Read the model definition and answer for the solid it produces. Units are mm, in the model's axes. Coordinates: 2 decimals unless noted, no trailing zeros. Write each loop counter-clockwise with the first axis right and the second up, starting at its lowest first coordinate (ties: lowest second). Pieces come first, ordered by that corner, then holes. Notation, with made-up numbers: (86, 32) - (136, 32) arc R20 cw to (136, 38) - close; hole circle Ø6 at (-34.5, 5.25). An arc over 180 degrees is marked (long way). Use a Markdown table: item, result.
from build123d import *

# Parameters (mm, degrees)
BOSS_EXTRUDE1_DEPTH         = 2.54
F_48_0_076_DIAMETER_HOLE1_D = 1.9304


with BuildPart() as part:
    # Sketch1 → Boss-Extrude1 (new body)
    with BuildSketch(Plane.XY):
        with BuildLine():
            Line((-1.523739013, -6.254008737), (3.199990263, -6.407247691))
            ThreePointArc((3.199990263, -6.407247691), (4.013460409, -6.008075165), (4.137562895, -5.110483411))
            add(Edge.make_bspline(
                [(4.137562895, -5.110483411), (3.751708737, -4.057424722), (1.960352922, -2.838406427), (0.682892057, -0.893226264), (0.419560202, 0.841832203), (0.235366214, 2.465138109), (0.366891085, 3.681965276), (0.493851252, 4.296654744)],
                knots=[0, 0, 0, 0, 0.339614963, 0.543785507, 0.644514611, 0.831601299, 1, 1, 1, 1], degree=3))
            add(Edge.make_bspline(
                [(-0.718288865, 6.33558287), (-0.121151201, 6.007229545), (0.640025429, 5.004370625), (0.493851252, 4.296654744)],
                knots=[0, 0, 0, 0, 1, 1, 1, 1], degree=3))
            ThreePointArc((-0.718288865, 6.33558287), (-1.649329968, 6.716784948), (-2.655033, 6.743505128))
            Line((-2.655033, 6.743505128), (-5.069160306, 6.367615902))
            ThreePointArc((-5.069160306, 6.367615902), (-5.974847558, 5.745610239), (-6.05644367, 4.64993578))
            add(Edge.make_bspline(
                [(-6.05644367, 4.64993578), (-5.472575235, 2.247634521), (-3.140324972, 0.9129092), (-2.564431384, -2.647350002), (-2.677357403, -4.146707908), (-2.496094371, -5.385625532)],
                knots=[0, 0, 0, 0, 0.493395358, 0.716015145, 1, 1, 1, 1], degree=3))
            ThreePointArc((-2.496094371, -5.385625532), (-2.167559601, -5.996334743), (-1.523739013, -6.254008737))
        make_face()
    extrude(amount=BOSS_EXTRUDE1_DEPTH)

    # #48 (0.076) Diameter Hole1 (through all)
    with Locations(Plane.XY.offset(2.54)):
        with Locations((1.811202951, -5.091527006)):
            Hole(F_48_0_076_DIAMETER_HOLE1_D / 2)


solid = part.part
(1) Straight lines are drawn through the part: L1, parallel to Y at x = 1.25, z = 0.3; L2, parallel to X at y = -5.25, z = 2.05; L3, parallel to Y at x = -4.5, z = 1.5. For each, find the intervals that lie inside material, in ascending order.
Report:
| item | result |
|---|---|
| L1 | y = -6.34 to -5.88, -4.31 to -1.69 |
| L2 | x = -2.52 to 0.86, 2.76 to 4.18 |
| L3 | y = 1.71 to 6.46 |
(2) The mould has two halves that part along Y. Classify faces 1 (the cylindrical face through (1.29, -4.28, 1.25)), 2 (the cylindrical face through (-5.967, 5.759, 1.252)), 3 (the flat face through (-1, 0, 0)), 4 (the cylindrical face through (-2.175, -5.99, 1.252)): pulls with the +Y half, pulls with the -Y half, needs draft (parallel to the pull), parting line crosses it, or undercut.
Report:
| item | result |
|---|---|
| face 1 | undercut |
| face 2 | parting line crosses it |
| face 3 | needs draft |
| face 4 | pulls with the -Y half |
(3) This flat-tipped pin is pushed along its axis until it touches: P1, Ø2, axis at x = -2, y = 5, coming from the -Z side. Where does it stop, or does it pass through?
Report:
| item | result |
|---|---|
| P1 | stops at z = 0 |
(4) A cutting plane is placed at A-A, the plane x = -1.75. Write down the section's boundary in (y, z), and give its area (3 significant figures).
Report:
| item | result |
|---|---|
| outline | (-6.22, 0) - (6.74, 0) - (6.74, 2.54) - (-6.22, 2.54) - close |
| area | 32.9 mm² |
